Model file for the job. Use its own axes, mm. A direction names the side the tool comes from. Give positions to 0.01 mm unless a question says otherwise; leave off trailing zeros. Loops run counter-clockwise (first coordinate to the right, second up) from the corner with the lowest first, then second, coordinate; pieces in that order, holes last. Notation, with made-up numbers: M 34,69.5 L 84,69.5 A26 cw 84,85.5 Z; hole C 58,35 d7. An arc over 180 degrees is marked long. Answer in a Markdown table with one row per item.
```python
from build123d import *

# Parameters (mm, degrees)
SKETCH1_R           = 1.25
SKETCH1_R_2         = 1.5
BOSS_EXTRUDE1_DEPTH = 3


with BuildPart() as part:
    # Sketch1 → Boss-Extrude1 (new body)
    with BuildSketch(Plane.XY):
        Polygon((-31.401650429, 13.901650429), (-25.938490407, 13.901650429), (-25.938490407, -26.201638424), (-31.401650429, -26.201638424), (-36.223809579, -26.201638424), (-36.223809579, -20.354504277), (-31.401650429, -18.062129594), align=None)
        with Locations((-28.670070418, 11.170070418)):
            Circle(SKETCH1_R, mode=Mode.SUBTRACT)
        with Locations((-28.670070418, -11.879929582)):
            Circle(SKETCH1_R, mode=Mode.SUBTRACT)
        with Locations((-31.779993959, -22.69389364)):
            Circle(SKETCH1_R_2, mode=Mode.SUBTRACT)
    extrude(amount=BOSS_EXTRUDE1_DEPTH)


solid = part.part
```
(1) Wall check: L1, parallel to X at y = 12.5, z = 0.45; L2, parallel to Y at x = -29.75, z = 0.9; L3, parallel to Y at x = -30.75, z = 2.45. Give the ranges that are in metal, low to high.
Established:
| item | result |
|---|---|
| L1 | x = -31.4 to -25.94 |
| L2 | y = -26.2 to -12.51, -11.25 to 10.54, 11.8 to 13.9 |
| L3 | y = -26.2 to -23.78, -21.6 to 13.9 |
(2) Saw through at A-A, the plane x = -28.75. Give the cut face in (y, z).
Established:
| item | result |
|---|---|
| outline | M -26.2,0 L -13.13,0 L -13.13,3 L -26.2,3 Z; M -10.63,0 L 9.92,0 L 9.92,3 L -10.63,3 Z; M 12.42,0 L 13.9,0 L 13.9,3 L 12.42,3 Z |
(3) Saw through at C-C, the plane x = -31.75. Give the cut face in (y, z), and give its area (3 significant figures).
Established:
| item | result |
|---|---|
| outline | M -26.2,0 L -24.19,0 L -24.19,3 L -26.2,3 Z; M -21.19,0 L -18.23,0 L -18.23,3 L -21.19,3 Z |
| area | 14.9 mm2 |
(4) Saw through at D-D, the plane y = -1. Give the cut face in (x, z).
Established:
| item | result |
|---|---|
| outline | M -31.4,0 L -25.94,0 L -25.94,3 L -31.4,3 Z |
(5) Mould opens along X. For faces 3 (the flat face through (-29, 13.902, 1)), 4 (the flat face through (-25.938, -6, 1)), 5 (the cylindrical face through (-32.886, -21.68, 1.479)), 6 (the flat face through (-33.846, -19.224, 1.479)) say: pulls with the +X half, pulls with the -X half, needs draft (parallel to the pull), parting line crosses it, or undercut.
Established:
| item | result |
|---|---|
| face 3 | needs draft |
| face 4 | pulls with the +X half |
| face 5 | undercut |
| face 6 | pulls with the -X half |
(6) Saw through at B-B, the plane z = 1.35. Give the cut face in (x, y), and give its area (3 significant figures).
Established:
| item | result |
|---|---|
| outline | M -36.22,-26.2 L -25.94,-26.2 L -25.94,13.9 L -31.4,13.9 L -31.4,-18.06 L -36.22,-20.35 Z; hole C -31.78,-22.69 d3; hole C -28.67,-11.88 d2.5; hole C -28.67,11.17 d2.5 |
| area | 236 mm2 |
(7) Flat gauge pins, fed straight in: P1, Ø0.9, axis at y = -7.5, z = 1, coming from the -X side; P2, Ø4, axis at x = -32, y = 0, coming from the -Z side. Where does each tip first touch, or does it go through?
Established:
| item | result |
|---|---|
| P1 | stops at x = -31.4 |
| P2 | stops at z = 0 |
(8) Which spindle directions (+Z, -Z, +X, -X, +Y, -Y) get a long thin tool onto all of the face, cutting with end or side? Do faces 1 (the flat face through (-31.402, -2, 1)), 2 (the cylindrical face through (-27.515, -12.359, 1.479)). Say none if no direction does.
Established:
| item | result |
|---|---|
| face 1 | +Z, -Z, -X, +Y |
| face 2 | +Z, -Z |
